Autodesk Inventor part; units mm, degrees
ref_plane "Start Plane" through (0, 0, 0) normal (0, 0, 1) x (1, 0, 0)
ref_plane "End Plane" through (0, 0, 2565.4) normal (0, 0, 1) x (1, 0, 0)
ref_plane "Work Plane4" through (1219.169, 0, 0) normal (0, 0, -1) x (-1, 0, 0)
ref_plane "Start Plane" through (0, 0, 0) normal (0, 0, 1) x (1, 0, 0)
ref_plane "End Plane" through (0, 0, 2565.4) normal (0, 0, 1) x (1, 0, 0)
sketch "Sketch" plane through (0, 0, 0) normal (0, 0, 1) x (1, 0, 0)
  line L0 (-25.4, -31.75) -> (-25.4, 31.75)
  line L1 (-19.05, 38.1) -> (19.05, 38.1)
  line L2 (25.4, 31.75) -> (25.4, -31.75)
  line L3 (19.05, -38.1) -> (-19.05, -38.1)
  arc A0 (-25.4, -31.75) -> (-19.05, -38.1) centre (-19.05, -31.75) ccw
  arc A1 (-19.05, 38.1) -> (-25.4, 31.75) centre (-19.05, 31.75) ccw
  arc A2 (25.4, 31.75) -> (19.05, 38.1) centre (19.05, 31.75) ccw
  arc A3 (19.05, -38.1) -> (25.4, -31.75) centre (19.05, -31.75) ccw
  arc A4 (-19.05, 34.925) -> (-22.225, 31.75) centre (-19.05, 31.75) ccw
  line L4 (-19.05, 34.925) -> (19.05, 34.925)
  arc A5 (22.225, 31.75) -> (19.05, 34.925) centre (19.05, 31.75) ccw
  line L5 (22.225, 31.75) -> (22.225, -31.75)
  arc A6 (19.05, -34.925) -> (22.225, -31.75) centre (19.05, -31.75) ccw
  line L6 (19.05, -34.925) -> (-19.05, -34.925)
  arc A7 (-22.225, -31.75) -> (-19.05, -34.925) centre (-19.05, -31.75) ccw
  line L7 (-22.225, -31.75) -> (-22.225, 31.75)
  line L8 (0, 55.1812) -> (0, -55.1812) construction
  line L9 (-37.4012, 0) -> (37.4012, 0) construction
  dimension "d10" = 76.2
  dimension "d11" = 50.8
  dimension "d12" = 3.175
  dimension "d15" = 38.1
  dimension "d16" = 25.4
  dimension "d17" = 6.35
extrude "Body" add sketch "Sketch" along normal up to surface (2565.4 mm away) from surface at 0
sketch "Sketch3" plane through (0, 0, 0) normal (0, 0, 1) x (1, 0, 0)
  line L0 (0, 0) -> (10, 0)
ref_plane "Work Plane3" through (0, 0, 0) normal (0, -1, 0) x (1, 0, 0)
ref_plane "Work Plane4" through (1219.169, 0, 0) normal (0, 0, -1) x (-1, 0, 0)
split "Split1" plane through (1219.169, 0, 0) removes the side toward (0, 0, -1)
ref_plane "Work Plane5" through (-25.4, 0, 2565.4) normal (0, 0, 1) x (1, 0, 0)
split "Split2" plane through (-25.4, 0, 2565.4) removes the side toward (0, 0, 1)
sketch "Sketch4" plane through (0, 0, 0) normal (0, -1, 0) x (1, 0, 0)
  line L0 (-2, 0) -> (12, 0)
  line L1 (-2, 2565.4) -> (12, 2565.4)
  dimension "d19" = 2565.4
equation "\"d10\" = G_H"
equation "\"d11\" = G_W"
equation "\"d12\" = G_T"
equation "\"d15\" = 0.5 * d10"
equation "\"d16\" = 0.5 * d11"
equation "\"d17\" = G_IR"
equation "\"d3\" = G_L"
equation "\"G_W\" = 50.8"
equation "\"G_H\" = 76.2"
equation "\"G_T\" = 3.175"
equation "\"G_IR\" = 6.35"
equation "\"G_L\" = d19"
equation "\"G_OFFSET_START\" = 0"
equation "\"G_OFFSET_END\" = 0"
equation "\"d14\" = G_OFFSET_END + B_L"
equation "\"B_L\" = 2565.4"
properties part number "AISC - 3 x 2 x 1/8 - 101" material "Steel, Mild"
Model file for the job. Use its own axes, mm. A direction names the side the tool comes from. Coordinates: 2 decimals unless noted, no trailing zeros. Write each loop counter-clockwise with the first axis right and the second up, starting at its lowest first coordinate (ties: lowest second). Pieces come first, ordered by that corner, then holes. Notation, with made-up numbers: (68, 60.25) - (125, 60.25) arc R12 ccw to (125, 72.25) - close; hole circle Ø3 at (59.5, -37). An arc over 180 degrees is marked (long way). One line per item, written item: value. Start each with the question number.
1. Probe line 1 (X direction, y = 4.5, z = 2006.5) (3 decimals); line 2 (Y direction, x = 8, z = 2367) (3 decimals); line 3 (X direction, y = -34.5, z = 802.5). List the from-to ranges inside material, lowest first. Write a range as from..to.
2. Slice it at C-C (x = -8). Write the cut outline in (y, z) (3 decimals).
3. Mould opens along Y. For faces 3 (the flat face through (-22.225, 0, 1265)), 4 (the flat face through (-23, 0, 2565.4)) say: released by +Y, released by -Y, zero draft, split by the parting line, or undercut.
4. Slice it at A-A (y = 19). Write the cut outline in (x, z) (3 decimals).
5. Slice it at B-B (z = 543.5). Write the cut outline in (x, y) (3 decimals).
6. Tool access for faces 1 (the flat face through (25.4, 0, 1265)), 2 (the flat face through (22.225, 0, 1265)): list every direction of +Z, -Z, +X, -X, +Y, -Y with a clear straight run to the whole face (end or side of a thin tool).
Answers below:
1. line 1: x = -25.4..-22.225, 22.225..25.4
1. line 2: y = -38.1..-34.925, 34.925..38.1
1. line 3: x = -24.77..-20.64, 20.64..24.77
2. outline: (-38.1, 0) - (-34.925, 0) - (-34.925, 2565.4) - (-38.1, 2565.4) - close; (34.925, 0) - (38.1, 0) - (38.1, 2565.4) - (34.925, 2565.4) - close
3. face 3: undercut
3. face 4: zero draft
4. outline: (-25.4, 0) - (-22.225, 0) - (-22.225, 2565.4) - (-25.4, 2565.4) - close; (22.225, 0) - (25.4, 0) - (25.4, 2565.4) - (22.225, 2565.4) - close
5. outline: (-25.4, -31.75) arc R6.35 ccw to (-19.05, -38.1) - (19.05, -38.1) arc R6.35 ccw to (25.4, -31.75) - (25.4, 31.75) arc R6.35 ccw to (19.05, 38.1) - (-19.05, 38.1) arc R6.35 ccw to (-25.4, 31.75) - close; hole (-22.225, -31.75) arc R3.175 ccw to (-19.05, -34.925) - (19.05, -34.925) arc R3.175 ccw to (22.225, -31.75) - (22.225, 31.75) arc R3.175 ccw to (19.05, 34.925) - (-19.05, 34.925) arc R3.175 ccw to (-22.225, 31.75) - close
6. face 1: +Z, -Z, +X, +Y, -Y
6. face 2: +Z, -Z
